Can you work these out from the model? Positions are in its coordinate system, mm. A direction names the side the tool comes from. Give positions to 0.01 mm unless a question says otherwise; leave off trailing zeros. Write each loop counter-clockwise with the first axis right and the second up, starting at its lowest first coordinate (ties: lowest second). Pieces come first, ordered by that corner, then holes.
from build123d import *

# Parameters (mm, degrees)
SKETCH_1_W          = 23
SKETCH_1_H          = 22
SKETCH_1_R          = 1.5
EXTRUDE_1_DEPTH     = 30
SKETCH_2_W          = 16
SKETCH_2_H          = 15
CUT_EXTRUDE_1_DEPTH = 34.959534744
FILLET_1_R          = 1


with BuildPart() as part:
    # 草图1 → 凸台-拉伸1 (new body)
    with BuildSketch(Plane.XY):
        Rectangle(SKETCH_1_W, SKETCH_1_H)
        with Locations((-8, 7.5)):
            Circle(SKETCH_1_R, mode=Mode.SUBTRACT)
        with Locations((8, 7.5)):
            Circle(SKETCH_1_R, mode=Mode.SUBTRACT)
        with Locations((-8, -7.5)):
            Circle(SKETCH_1_R, mode=Mode.SUBTRACT)
        with Locations((8, -7.5)):
            Circle(SKETCH_1_R, mode=Mode.SUBTRACT)
    extrude(amount=EXTRUDE_1_DEPTH)

    # 草图2 → 切除-拉伸1 (cut, through all)
    with BuildSketch(Plane.XY.offset(30)):
        with Locations((-3.5, -3.5)):
            Rectangle(SKETCH_2_W, SKETCH_2_H)
    extrude(amount=-CUT_EXTRUDE_1_DEPTH, mode=Mode.SUBTRACT)

    # 圆角1
    fillet_1_edges = [part.edges().sort_by_distance(p)[0] for p in [
        (-11.5, 4, 15),
        (4.5, 4, 15),
        (4.5, -11, 15),
        (11.5, -11, 15),
        (-11.5, 11, 15),
        (11.5, 11, 15),
    ]]
    fillet(fillet_1_edges, radius=FILLET_1_R)


solid = part.part
(1) Imagine slicing it at D-D, the plane z = 14.75. Write out the boundary of the cut face in (x, y).
Returned:
outline: (-11.5, 5) arc R1 ccw to (-10.5, 4) - (3.5, 4) arc R1 cw to (4.5, 3) - (4.5, -10) arc R1 ccw to (5.5, -11) - (10.5, -11) arc R1 ccw to (11.5, -10) - (11.5, 10) arc R1 ccw to (10.5, 11) - (-10.5, 11) arc R1 ccw to (-11.5, 10) - close; hole circle Ø3 at (-8, 7.5); hole circle Ø3 at (8, -7.5); hole circle Ø3 at (8, 7.5)
(2) If I drill on L1, parallel to Y at x = 8, z = 3.25; L2, parallel to Y at x = -8, z = 13; L3, parallel to X at y = 0.5, z = 13.25, over which ranges is the centre line in solid material (lowest first)?
Returned:
L1: y = -11 to -9, -6 to 6, 9 to 11
L2: y = 4 to 6, 9 to 11
L3: x = 4.5 to 11.5
(3) Imagine slicing it at C-C, the plane y = 7.5. Write out the boundary of the cut face in (x, z).
Returned:
outline: (-11.5, 0) - (-9.5, 0) - (-9.5, 30) - (-11.5, 30) - close; (-6.5, 0) - (6.5, 0) - (6.5, 30) - (-6.5, 30) - close; (9.5, 0) - (11.5, 0) - (11.5, 30) - (9.5, 30) - close
(4) For faces 1 (the face through (6.8, 6.6, 14.8)), 2 (the face through (4.5, -4, 15)), which set-ups out of +Z, -Z, +X, -X, +Y, -Y let a thin tool reach every point of the face, with its end or its side?
Returned:
face 1: +Z, -Z
face 2: +Z, -Z, -X, -Y
(5) Imagine slicing it at B-B, the plane x = -8. Write out the boundary of the cut face in (y, z), plus the area to 3 significant figures.
Returned:
outline: (4, 0) - (6, 0) - (6, 30) - (4, 30) - close; (9, 0) - (11, 0) - (11, 30) - (9, 30) - close
area: 120 mm2
(6) Imagine slicing it at A-A, the plane x = 8. Write out the boundary of the cut face in (y, z).
Returned:
outline: (-11, 0) - (-9, 0) - (-9, 30) - (-11, 30) - close; (-6, 0) - (6, 0) - (6, 30) - (-6, 30) - close; (9, 0) - (11, 0) - (11, 30) - (9, 30) - close
(7) Will these pins go through, and if not, where does the flat tip stop? P1, Ø4, axis at y = -7, z = 16.5, coming from the -X side; P2, Ø2.5, axis at x = -8, y = 7.5, coming from the +Z side.
Returned:
P1: stops at x = 4.5
P2: passes through
(8) If we mould it in two halves opening along X, with no side actions, what happens to faces 3 (the face through (2, 5, 0)), 4 (the face through (-8, 6, 15)), 5 (the face through (6.8, -8.4, 14.8)), 6 (the face through (11.215, -10.699, 15.21))? For each: +X half, -X half, draft (parallel to the pull), parting line (faces both ways), or undercut.
Returned:
face 3: draft
face 4: undercut
face 5: undercut
face 6: +X half
